Part model, mm, in its own coordinate system. Round coordinates to 2 decimals unless told otherwise and drop trailing zeros. Order: outer loops, then holes, each group sorted by start corner. A loop starts at its lowest first (then second) coordinate and runs counter-clockwise, first axis right, second up. Notation, with made-up numbers: M 28.5,46 L 65.5,46 A8 ccw 65.5,59 Z; hole C -34.75,20 d4. An arc over 180 degrees is marked long. One line per question, with ' | ' between items.
Autodesk Inventor part; units mm, degrees
ref_plane "YZ Plane" through (0, 0, 0) normal (1, 0, 0) x (0, 1, 0)
ref_plane "XZ Plane" through (0, 0, 0) normal (0, 1, 0) x (-1, 0, 0)
ref_plane "XY Plane" through (0, 0, 0) normal (0, 0, 1) x (1, 0, 0)
sketch "Sketch1" plane through (0, 0, 0) normal (0, 0, 1) x (1, 0, 0)
  line L0 (-39.7468, 54.4174) -> (-39.7468, -52.4226)
  line L1 (-39.7468, -52.4226) -> (-26.9468, -52.4226)
  line L2 (-26.9468, -52.4226) -> (-26.9468, -70.2026)
  line L3 (-26.9468, -70.2026) -> (5.6532, -70.2026)
  line L4 (5.6532, -70.2026) -> (5.6532, -52.4226)
  line L5 (5.6532, -52.4226) -> (18.4532, -52.4226)
  line L6 (18.4532, -52.4226) -> (18.4532, 54.4174)
  line L7 (18.4532, 54.4174) -> (5.6532, 54.4174)
  line L8 (5.6532, 54.4174) -> (5.6532, 72.1974)
  line L9 (5.6532, 72.1974) -> (-26.9468, 72.1974)
  line L10 (-26.9468, 72.1974) -> (-26.9468, 54.4174)
  line L11 (-39.7468, 54.4174) -> (-26.9468, 54.4174)
  line L12 (-23.8279, 76.1974) -> (9.6532, 76.1974)
  line L13 (9.6532, 76.1974) -> (9.6532, 58.4174)
  line L14 (9.6532, 58.4174) -> (22.4532, 58.4174)
  line L15 (22.4532, 58.4174) -> (22.4532, -56.4226)
  line L16 (22.4532, -56.4226) -> (9.6532, -56.4226)
  line L17 (9.6532, -56.4226) -> (9.6532, -74.2026)
  line L18 (9.6532, -74.2026) -> (-30.9468, -74.2026)
  line L19 (-30.9468, -74.2026) -> (-30.9468, -56.4226)
  line L20 (-30.9468, -56.4226) -> (-43.7468, -56.4226)
  line L21 (-43.7468, -56.4226) -> (-43.7468, 58.4174)
  line L22 (-43.7468, 58.4174) -> (-30.9468, 58.4174)
  line L23 (-30.9468, 76.1974) -> (-23.8279, 76.1974)
  line L24 (-30.9468, 58.4174) -> (-30.9468, 76.1974)
  point P0 (0, 0)
  dimension "d0" = 106.84
  dimension "d1" = 142.4
  dimension "d2" = 17.78
  dimension "d3" = 17.78
  dimension "d4" = 32.6
  dimension "d5" = 12.8
  dimension "d6" = 12.8
  dimension "d7" = 4
  dimension "d8" = 4
  dimension "d9" = 4
  dimension "d10" = 4
  dimension "d11" = 4
  dimension "d12" = 4
  dimension "d13" = 4
  dimension "d14" = 4
  dimension "d15" = 4
sketch "Sketch2" plane through (0, 0, 0) normal (0, 0, 1) x (1, 0, 0)
  circle A0 centre (-4.4728, 32.0701) radius 4
  circle A1 centre (-16.4728, 32.0701) radius 4
  circle A2 centre (-4.4728, 20.0701) radius 4
  circle A3 centre (-16.4728, 20.0701) radius 4
  circle A4 centre (-4.4728, 8.0701) radius 4
  circle A5 centre (-16.4728, 8.0701) radius 4
  circle A6 centre (-4.4728, -3.9299) radius 4
  circle A7 centre (-16.4728, -15.9299) radius 4
  circle A8 centre (-4.4728, -15.9299) radius 4
  circle A9 centre (-16.4728, -3.9299) radius 4
  circle A10 centre (-4.4728, -27.9299) radius 4
  circle A11 centre (-16.4728, -27.9299) radius 4
  point P0 (0, 0)
  dimension "d22" = 8
  dimension "d27" = 8
  dimension "d30" = 8
  dimension "d34" = 8
  dimension "d38" = 8
  dimension "d42" = 8
  dimension "d59" = 12
  dimension "d63" = 12
  dimension "d67" = 12
  dimension "d70" = 12
  dimension "d71" = 12
  dimension "d75" = 12
  dimension "d93" = 12
  dimension "d94" = 0
  dimension "d97" = 0
  dimension "d98" = 12
  dimension "d102" = 0
  dimension "d103" = 12
extrude "Extrusion1" add sketch "Sketch1" along normal blind 6 contours L11 L10 L9 L8 L7 L6 L5 L4 L3 L2 L1 L0
extrude "Extrusion2" add sketch "Sketch1" along normal blind 4
extrude "Extrusion3" cut sketch "Sketch2" along normal blind 12
properties part number "rib"
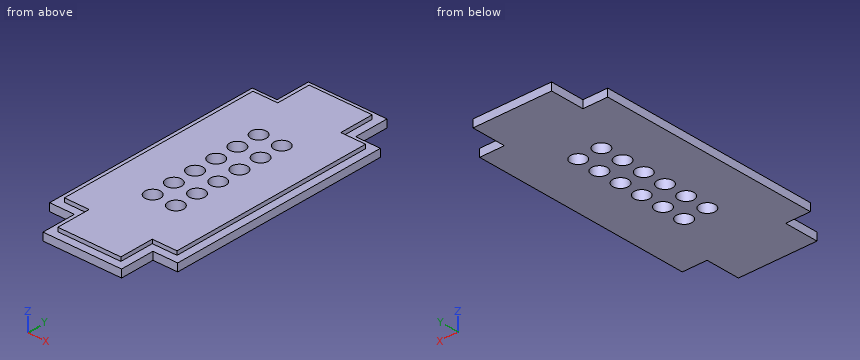
1) Saw through at C-C (x = -34). List the corners of the cut face in (y, z).
The answers:
outline: M -56.42,0 L 58.42,0 L 58.42,4 L 54.42,4 L 54.42,6 L -52.42,6 L -52.42,4 L -56.42,4 Z
2) Saw through at A-A (y = -49.5). List the corners of the cut face in (x, z).
The answers:
outline: M -43.75,0 L 22.45,0 L 22.45,4 L 18.45,4 L 18.45,6 L -39.75,6 L -39.75,4 L -43.75,4 Z
3) Drop flat-ended pins along their axis: pin 1 (1 mm diameter, centred on x = -4, z = 5, fed in from +Y); pin 2 (1 mm diameter, centred on y = -24.5, z = 5, fed in from -X); pin 3 (5 mm diameter, centred on x = -16.47, y = 20.07, fed in from +Z); pin 4 (3 mm diameter, centred on y = 64, z = 2, fed in from +X). Give the stop position or say it passes through.
The answers:
pin 1: stops at y = 72.2 | pin 2: stops at x = -39.75 | pin 3: passes through | pin 4: stops at x = 9.65
4) Saw through at B-B (z = 5.1). Give the number of separate pieces and of enclosed holes in the cut face, plus the area to 3 significant figures.
The answers:
separate pieces: 1 | enclosed holes: 12 | area: 6,770 mm²
5) Saw through at D-D (y = 6). List the corners of the cut face in (x, z).
The answers:
outline: M -43.75,0 L -19.9,0 L -19.9,6 L -39.75,6 L -39.75,4 L -43.75,4 Z; M -13.05,0 L -7.9,0 L -7.9,6 L -13.05,6 Z; M -1.05,0 L 22.45,0 L 22.45,4 L 18.45,4 L 18.45,6 L -1.05,6 Z
6) Probe line 1 (X direction, y = 31, z = 0.75); line 2 (X direction, y = 31.5, z = 0.8); line 3 (Y direction, x = 12.5, z = 3.7). List the from-to ranges inside material, lowest first. Write a range as [from, to].
The answers:
line 1: x = [-43.75, -20.33], [-12.62, -8.33], [-0.62, 22.45] | line 2: x = [-43.75, -20.43], [-12.51, -8.43], [-0.51, 22.45] | line 3: y = [-56.42, 58.42]
